The listing builds one solid part. Answer for the finished solid, in the listing's coordinates (mm). A direction names the side the tool comes from. Coordinates: 2 decimals unless noted, no trailing zeros. Write each loop counter-clockwise with the first axis right and the second up, starting at its lowest first coordinate (ties: lowest second). Pieces come first, ordered by that corner, then holes.
```python
from build123d import *

# Parameters (mm, degrees)
SKETCH1_W           = 86
SKETCH1_H           = 86
SKETCH1_R           = 3
BOSS_EXTRUDE1_DEPTH = 3
SKETCH1_4_W         = 3
SKETCH1_4_H         = 84
SKETCH1_4_W_2       = 84
SKETCH1_4_H_2       = 3
BOSS_EXTRUDE3_DEPTH = 23
FILLET1_R           = 2
CUT_EXTRUDE1_REACH  = 94
SKETCH2_R           = 1.5
CUT_EXTRUDE2_REACH  = 94
SKETCH3_R           = 1.5
CUT_EXTRUDE3_REACH  = 94
SKETCH4_R           = 1.5
CUT_EXTRUDE4_REACH  = 94
SKETCH5_R           = 1.5


with BuildPart() as part:
    # Sketch1 → Boss-Extrude1 (new body)
    with BuildSketch(Plane.XY):
        with Locations((-20.693877551, 22.317784257)):
            Rectangle(SKETCH1_W, SKETCH1_H)
        with Locations((-56.193877551, -13.182215743)):
            Circle(SKETCH1_R, mode=Mode.SUBTRACT)
        with Locations((14.806122449, -13.182215743)):
            Circle(SKETCH1_R, mode=Mode.SUBTRACT)
        with Locations((14.806122449, 57.817784257)):
            Circle(SKETCH1_R, mode=Mode.SUBTRACT)
        with Locations((-56.193877551, 57.817784257)):
            Circle(SKETCH1_R, mode=Mode.SUBTRACT)
    extrude(amount=BOSS_EXTRUDE1_DEPTH)

    # Sketch1_4 → Boss-Extrude3 (add)
    with BuildSketch(Plane.XY):
        with Locations((-65.193877551, 22.317784257)):
            Rectangle(SKETCH1_4_W, SKETCH1_4_H)
        with Locations((-20.693877551, 66.817784257)):
            Rectangle(SKETCH1_4_W_2, SKETCH1_4_H_2)
        with Locations((-20.693877551, -22.182215743)):
            Rectangle(SKETCH1_4_W_2, SKETCH1_4_H_2)
        with Locations((23.806122449, 22.317784257)):
            Rectangle(SKETCH1_4_W, SKETCH1_4_H)
    extrude(amount=BOSS_EXTRUDE3_DEPTH)

    # Fillet1
    fillet1_edges = [part.edges().sort_by_distance(p)[0] for p in [
        (-66.693877551, 22.317784257, 0),
        (-20.693877551, 68.317784257, 0),
        (-20.693877551, -23.682215743, 0),
        (25.306122449, 22.317784257, 0),
    ]]
    fillet(fillet1_edges, radius=FILLET1_R)

    # Sketch2 → Cut-Extrude1 (cut, up to next)
    with BuildSketch(Plane.ZY.offset(66.693877551), mode=Mode.PRIVATE) as cut_extrude1_sk1:
        with Locations((12, -16.682215743)):
            Circle(SKETCH2_R)
    cut_extrude1_tool1 = extrude(cut_extrude1_sk1.sketch, amount=-CUT_EXTRUDE1_REACH, mode=Mode.PRIVATE) & part.part
    add(cut_extrude1_tool1.solids().sort_by_distance((-66.693878, -16.682216, 12))[0], mode=Mode.SUBTRACT)
    # Sketch2 → Cut-Extrude1 (cut, up to next)
    with BuildSketch(Plane.ZY.offset(66.693877551), mode=Mode.PRIVATE) as cut_extrude1_sk2:
        with Locations((18, -16.682215743)):
            Circle(SKETCH2_R)
    cut_extrude1_tool2 = extrude(cut_extrude1_sk2.sketch, amount=-CUT_EXTRUDE1_REACH, mode=Mode.PRIVATE) & part.part
    add(cut_extrude1_tool2.solids().sort_by_distance((-66.693878, -16.682216, 18))[0], mode=Mode.SUBTRACT)
    # Sketch2 → Cut-Extrude1 (cut, up to next)
    with BuildSketch(Plane.ZY.offset(66.693877551), mode=Mode.PRIVATE) as cut_extrude1_sk3:
        with Locations((12, 61.317784257)):
            Circle(SKETCH2_R)
    cut_extrude1_tool3 = extrude(cut_extrude1_sk3.sketch, amount=-CUT_EXTRUDE1_REACH, mode=Mode.PRIVATE) & part.part
    add(cut_extrude1_tool3.solids().sort_by_distance((-66.693878, 61.317784, 12))[0], mode=Mode.SUBTRACT)
    # Sketch2 → Cut-Extrude1 (cut, up to next)
    with BuildSketch(Plane.ZY.offset(66.693877551), mode=Mode.PRIVATE) as cut_extrude1_sk4:
        with Locations((18, 61.317784257)):
            Circle(SKETCH2_R)
    cut_extrude1_tool4 = extrude(cut_extrude1_sk4.sketch, amount=-CUT_EXTRUDE1_REACH, mode=Mode.PRIVATE) & part.part
    add(cut_extrude1_tool4.solids().sort_by_distance((-66.693878, 61.317784, 18))[0], mode=Mode.SUBTRACT)

    # Sketch3 → Cut-Extrude2 (cut, up to next)
    with BuildSketch(Plane.XZ.offset(23.682215743), mode=Mode.PRIVATE) as cut_extrude2_sk1:
        with Locations((18.306122449, 12)):
            Circle(SKETCH3_R)
    cut_extrude2_tool1 = extrude(cut_extrude2_sk1.sketch, amount=-CUT_EXTRUDE2_REACH, mode=Mode.PRIVATE) & part.part
    add(cut_extrude2_tool1.solids().sort_by_distance((18.306122, -23.682216, 12))[0], mode=Mode.SUBTRACT)
    # Sketch3 → Cut-Extrude2 (cut, up to next)
    with BuildSketch(Plane.XZ.offset(23.682215743), mode=Mode.PRIVATE) as cut_extrude2_sk2:
        with Locations((18.306122449, 18)):
            Circle(SKETCH3_R)
    cut_extrude2_tool2 = extrude(cut_extrude2_sk2.sketch, amount=-CUT_EXTRUDE2_REACH, mode=Mode.PRIVATE) & part.part
    add(cut_extrude2_tool2.solids().sort_by_distance((18.306122, -23.682216, 18))[0], mode=Mode.SUBTRACT)
    # Sketch3 → Cut-Extrude2 (cut, up to next)
    with BuildSketch(Plane.XZ.offset(23.682215743), mode=Mode.PRIVATE) as cut_extrude2_sk3:
        with Locations((-59.693877551, 12)):
            Circle(SKETCH3_R)
    cut_extrude2_tool3 = extrude(cut_extrude2_sk3.sketch, amount=-CUT_EXTRUDE2_REACH, mode=Mode.PRIVATE) & part.part
    add(cut_extrude2_tool3.solids().sort_by_distance((-59.693878, -23.682216, 12))[0], mode=Mode.SUBTRACT)
    # Sketch3 → Cut-Extrude2 (cut, up to next)
    with BuildSketch(Plane.XZ.offset(23.682215743), mode=Mode.PRIVATE) as cut_extrude2_sk4:
        with Locations((-59.693877551, 18)):
            Circle(SKETCH3_R)
    cut_extrude2_tool4 = extrude(cut_extrude2_sk4.sketch, amount=-CUT_EXTRUDE2_REACH, mode=Mode.PRIVATE) & part.part
    add(cut_extrude2_tool4.solids().sort_by_distance((-59.693878, -23.682216, 18))[0], mode=Mode.SUBTRACT)

    # Sketch4 → Cut-Extrude3 (cut, up to next)
    with BuildSketch(Plane(origin=(25.306122449, 0, 0), x_dir=(0, 0, -1), z_dir=(1, 0, 0)), mode=Mode.PRIVATE) as cut_extrude3_sk1:
        with Locations((-12, 61.317784257)):
            Circle(SKETCH4_R)
    cut_extrude3_tool1 = extrude(cut_extrude3_sk1.sketch, amount=-CUT_EXTRUDE3_REACH, mode=Mode.PRIVATE) & part.part
    add(cut_extrude3_tool1.solids().sort_by_distance((25.306122, 61.317784, 12))[0], mode=Mode.SUBTRACT)
    # Sketch4 → Cut-Extrude3 (cut, up to next)
    with BuildSketch(Plane(origin=(25.306122449, 0, 0), x_dir=(0, 0, -1), z_dir=(1, 0, 0)), mode=Mode.PRIVATE) as cut_extrude3_sk2:
        with Locations((-18, 61.317784257)):
            Circle(SKETCH4_R)
    cut_extrude3_tool2 = extrude(cut_extrude3_sk2.sketch, amount=-CUT_EXTRUDE3_REACH, mode=Mode.PRIVATE) & part.part
    add(cut_extrude3_tool2.solids().sort_by_distance((25.306122, 61.317784, 18))[0], mode=Mode.SUBTRACT)
    # Sketch4 → Cut-Extrude3 (cut, up to next)
    with BuildSketch(Plane(origin=(25.306122449, 0, 0), x_dir=(0, 0, -1), z_dir=(1, 0, 0)), mode=Mode.PRIVATE) as cut_extrude3_sk3:
        with Locations((-12, -16.682215743)):
            Circle(SKETCH4_R)
    cut_extrude3_tool3 = extrude(cut_extrude3_sk3.sketch, amount=-CUT_EXTRUDE3_REACH, mode=Mode.PRIVATE) & part.part
    add(cut_extrude3_tool3.solids().sort_by_distance((25.306122, -16.682216, 12))[0], mode=Mode.SUBTRACT)
    # Sketch4 → Cut-Extrude3 (cut, up to next)
    with BuildSketch(Plane(origin=(25.306122449, 0, 0), x_dir=(0, 0, -1), z_dir=(1, 0, 0)), mode=Mode.PRIVATE) as cut_extrude3_sk4:
        with Locations((-18, -16.682215743)):
            Circle(SKETCH4_R)
    cut_extrude3_tool4 = extrude(cut_extrude3_sk4.sketch, amount=-CUT_EXTRUDE3_REACH, mode=Mode.PRIVATE) & part.part
    add(cut_extrude3_tool4.solids().sort_by_distance((25.306122, -16.682216, 18))[0], mode=Mode.SUBTRACT)

    # Sketch5 → Cut-Extrude4 (cut, up to next)
    with BuildSketch(Plane(origin=(0, 68.317784257, 0), x_dir=(1, 0, 0), z_dir=(0, 1, 0)), mode=Mode.PRIVATE) as cut_extrude4_sk1:
        with Locations((-59.693877551, -12)):
            Circle(SKETCH5_R)
    cut_extrude4_tool1 = extrude(cut_extrude4_sk1.sketch, amount=-CUT_EXTRUDE4_REACH, mode=Mode.PRIVATE) & part.part
    add(cut_extrude4_tool1.solids().sort_by_distance((-59.693878, 68.317784, 12))[0], mode=Mode.SUBTRACT)
    # Sketch5 → Cut-Extrude4 (cut, up to next)
    with BuildSketch(Plane(origin=(0, 68.317784257, 0), x_dir=(1, 0, 0), z_dir=(0, 1, 0)), mode=Mode.PRIVATE) as cut_extrude4_sk2:
        with Locations((-59.693877551, -18)):
            Circle(SKETCH5_R)
    cut_extrude4_tool2 = extrude(cut_extrude4_sk2.sketch, amount=-CUT_EXTRUDE4_REACH, mode=Mode.PRIVATE) & part.part
    add(cut_extrude4_tool2.solids().sort_by_distance((-59.693878, 68.317784, 18))[0], mode=Mode.SUBTRACT)
    # Sketch5 → Cut-Extrude4 (cut, up to next)
    with BuildSketch(Plane(origin=(0, 68.317784257, 0), x_dir=(1, 0, 0), z_dir=(0, 1, 0)), mode=Mode.PRIVATE) as cut_extrude4_sk3:
        with Locations((18.306122449, -18)):
            Circle(SKETCH5_R)
    cut_extrude4_tool3 = extrude(cut_extrude4_sk3.sketch, amount=-CUT_EXTRUDE4_REACH, mode=Mode.PRIVATE) & part.part
    add(cut_extrude4_tool3.solids().sort_by_distance((18.306122, 68.317784, 18))[0], mode=Mode.SUBTRACT)
    # Sketch5 → Cut-Extrude4 (cut, up to next)
    with BuildSketch(Plane(origin=(0, 68.317784257, 0), x_dir=(1, 0, 0), z_dir=(0, 1, 0)), mode=Mode.PRIVATE) as cut_extrude4_sk4:
        with Locations((18.306122449, -12)):
            Circle(SKETCH5_R)
    cut_extrude4_tool4 = extrude(cut_extrude4_sk4.sketch, amount=-CUT_EXTRUDE4_REACH, mode=Mode.PRIVATE) & part.part
    add(cut_extrude4_tool4.solids().sort_by_distance((18.306122, 68.317784, 12))[0], mode=Mode.SUBTRACT)


solid = part.part
```
(1) Find the intervals of material crossed by probe 1 along X at (y, z) = (66.55, 12); probe 2 along X at (y, z) = (27, 19.25); probe 3 along Y at (x, z) = (-34.5, 13.25), in increasing order.
(2) Section C-C, the plane y = -9 is taken. Write down the section's boundary in (x, z), plus the area to 3 significant figures.
(3) Section A-A, the plane z = 21.5 is taken. Write down the section's boundary in (x, y), plus the area to 3 significant figures.
(4) Which of the six approach directions +Z, -Z, +X, -X, +Y, -Y give full straight-line access (tool end or side, diameter ignored) to faces 4 (the cylindrical face through (23.827, 62.332, 13.106)), 5 (the flat face through (-63.694, 22, 13)), 6 (the flat face through (-21, -20.682, 13))?
(5) For a pull along X with two mould halves and no side action, classify faces 1 (the flat face through (-66.694, 22, 12)), 2 (the flat face through (25.306, 22, 12)), 3 (the cylindrical face through (-59.889, 66.839, 16.513)) as pulls with the +X half, pulls with the -X half, needs draft (parallel to the pull), parting line crosses it, or undercut.
(6) Each of these flat-tipped pins is pushed along its axis until it touches: pin 1 (0.9 mm diameter, centred on y = 66.5, z = 6.5, fed in from +X); pin 2 (3.5 mm diameter, centred on y = -22, z = 16, fed in from -X); pin 3 (2 mm diameter, centred on x = -11.5, y = 43.5, fed in from +Z). Where does it stop, or does it pass through?
(7) Section D-D, the plane x = -39.5 is taken. Write down the section's boundary in (y, z), plus the area to 3 significant figures.
(8) Section B-B, the plane x = 15.5 is taken. Write down the section's boundary in (y, z), plus the area to 3 significant figures.
Solution:
1. probe 1: x = -62.69 to -61.19, -58.19 to 16.81, 19.81 to 21.31
1. probe 2: x = -66.69 to -63.69, 22.31 to 25.31
1. probe 3: y = -23.68 to -20.68, 65.32 to 68.32
2. outline: (-66.69, 2) arc R2 ccw to (-64.69, 0) - (23.31, 0) arc R2 ccw to (25.31, 2) - (25.31, 23) - (22.31, 23) - (22.31, 3) - (-63.69, 3) - (-63.69, 23) - (-66.69, 23) - close
2. area: 394 mm2
3. outline: (-66.69, -19.68) - (-63.69, -19.68) - (-63.69, 64.32) - (-66.69, 64.32) - close; (-62.69, -23.68) - (21.31, -23.68) - (21.31, -20.68) - (-62.69, -20.68) - close; (-62.69, 65.32) - (21.31, 65.32) - (21.31, 68.32) - (-62.69, 68.32) - close; (22.31, -19.68) - (25.31, -19.68) - (25.31, 64.32) - (22.31, 64.32) - close
3. area: 1,010 mm2
4. face 4: +X, -X
4. face 5: +Z, +Y, -Y
4. face 6: +Z, +X, -X
5. face 1: pulls with the -X half
5. face 2: pulls with the +X half
5. face 3: undercut
6. pin 1: stops at x = 21.31
6. pin 2: stops at x = -62.69
6. pin 3: stops at z = 3
7. outline: (-23.68, 2) arc R2 ccw to (-21.68, 0) - (66.32, 0) arc R2 ccw to (68.32, 2) - (68.32, 23) - (65.32, 23) - (65.32, 3) - (-20.68, 3) - (-20.68, 23) - (-23.68, 23) - close
7. area: 394 mm2
8. outline: (-23.68, 2) arc R2 ccw to (-21.68, 0) - (-16.1, 0) - (-16.1, 3) - (-20.68, 3) - (-20.68, 23) - (-23.68, 23) - close; (-10.26, 0) - (54.9, 0) - (54.9, 3) - (-10.26, 3) - close; (60.74, 0) - (66.32, 0) arc R2 ccw to (68.32, 2) - (68.32, 23) - (65.32, 23) - (65.32, 3) - (60.74, 3) - close
8. area: 359 mm2
